```python
from build123d import *

# Parameters (mm, degrees)
SKETCH1_W           = 20.32
SKETCH1_H           = 26.081708108
SKETCH1_R           = 3.175
BOSS_EXTRUDE1_DEPTH = 22.098
SKETCH2_R           = 3.175
BOSS_EXTRUDE2_DEPTH = 5.08


with BuildPart() as part:
    # Sketch1 → Boss-Extrude1 (new body)
    with BuildSketch(Plane.XY):
        with Locations((-101.659894533, 115.530854428)):
            Rectangle(SKETCH1_W, SKETCH1_H)
        with Locations(Location((-104.04520642, 114, 0), (0, 0, 180))):
            Circle(SKETCH1_R, mode=Mode.SUBTRACT)
        with Locations(Location((-104.05047074, 124, 0), (0, 0, 180))):
            Circle(SKETCH1_R, mode=Mode.SUBTRACT)
    extrude(amount=BOSS_EXTRUDE1_DEPTH)

    # Sketch2 → Boss-Extrude2 (add)
    with BuildSketch(Plane(origin=(0, 102.490000374, 0), x_dir=(1, 0, 0), z_dir=(0, 1, 0))):
        Polygon((-96.663626928, 22.420429911), (-114.413437041, -43.822763256), (-93.559098452, -49.410666439), (-75.809288339, 16.832526727), align=None)
        with Locations(Location((-101.685366436, -38.029634252, 0), (0, 0, 270))):
            Circle(SKETCH2_R, mode=Mode.SUBTRACT)
        with Locations(Location((-88.537358944, 11.039397724, 0), (0, 0, 270))):
            Circle(SKETCH2_R, mode=Mode.SUBTRACT)
    extrude(amount=-BOSS_EXTRUDE2_DEPTH)


solid = part.part
```
The model under review builds one solid part; all positions refer to its coordinate system, in mm. A direction names the side the tool comes from. Coordinates: 2 decimals unless noted, no trailing zeros. Write each loop counter-clockwise with the first axis right and the second up, starting at its lowest first coordinate (ties: lowest second). Pieces come first, ordered by that corner, then holes. Notation, with made-up numbers: (52, -36) -> (67, -36) arc R35 cw to (67, 2) -> close; hole circle Ø4 at (-10, 12.5). An arc over 180 degrees is marked (long way). One line per item, written item: value. Start each with the question number.
Q1. To check wall thickness, follow probe 1 along X at (y, z) = (114, 16.5); probe 2 along Y at (x, z) = (-90.5, 36); probe 3 along Z at (x, y) = (-96.5, 116). State the ranges of each line that lie inside material, in increasing order.
Q2. Add section B-B, the plane z = 37. Give the boundary of the cut face in (x, y), then the cut area to 3 significant figures.
Q3. Clearance check with flat-ended pins moving along their axes: P1, Ø5, axis at x = -104.05, y = 124, coming from the -Z side; P2, Ø6.5, axis at y = 115, z = 9, coming from the -X side; P3, Ø12, axis at x = -90.5, y = 123.5, coming from the +Z side; P4, Ø5, axis at x = -93.5, y = 115, coming from the -Z side. State where each tip first meets the part, or that it passes through.
Q4. Add section D-D, the plane y = 107. Give the boundary of the cut face in (x, z), then the cut area to 3 significant figures.
Q5. For faces 1 (the face through (-100, 116, 0)), 2 (the face through (-100.732, 99.986, 41.058)), 3 (the face through (-108, 102.49, 8)), 4 (the face through (-91.5, 115, 11)), list the 3-axis set-ups (+Z, -Z, +X, -X, +Y, -Y) from which the entire face can be reached by the end or side of a thin tool; tool diameter is ignored.
Q6. The part is to be moulded in two halves that separate along Y. For faces 5 (the face through (-103.64, 120.85, 10.89)), 6 (the face through (-105.75, 111.32, 10.89)), 7 (the face through (-91, 102.49, 13)), 8 (the face through (-100, 116, 22.098)), say which applies: +Y half, -Y half, draft (parallel to the pull), parting line (faces both ways), or undercut.
Q7. Add section A-A, the plane y = 114. Give the boundary of the cut face in (x, z), then the cut area to 3 significant figures.
Q8. Add section C-C, the plane z = 10. Give the boundary of the cut face in (x, y) (3 decimals).
Response:
1. probe 1: -111.82 to -107.22, -100.87 to -91.5
1. probe 2: 97.41 to 102.49
1. probe 3: 0 to 22.1
2. outline: (-112.59, 97.41) -> (-104.69, 97.41) -> (-104.69, 102.49) -> (-112.59, 102.49) -> close; (-98.68, 97.41) -> (-90.23, 97.41) -> (-90.23, 102.49) -> (-98.68, 102.49) -> close
2. area: 83.0 mm²
3. P1: through
3. P2: x = -111.82
3. P3: z = 22.1
3. P4: z = 0
4. outline: (-111.82, 0) -> (-91.5, 0) -> (-91.5, 22.1) -> (-111.82, 22.1) -> close
4. area: 449 mm²
5. face 1: -Z, +X, -X, +Y
5. face 2: +Y, -Y
5. face 3: -Z, -X, -Y
5. face 4: +Z, -Z, +X, +Y
6. face 5: undercut
6. face 6: undercut
6. face 7: +Y half
6. face 8: draft
7. outline: (-111.82, 0) -> (-107.22, 0) -> (-107.22, 22.1) -> (-111.82, 22.1) -> close; (-100.87, 0) -> (-91.5, 0) -> (-91.5, 22.1) -> (-100.87, 22.1) -> close
7. area: 309 mm²
8. outline: (-111.82, 102.49) -> (-105.351, 102.49) -> (-105.351, 97.41) -> (-82.999, 97.41) -> (-82.999, 102.49) -> (-91.5, 102.49) -> (-91.5, 128.572) -> (-111.82, 128.572) -> close; hole circle Ø6.35 at (-104.05, 124); hole circle Ø6.35 at (-104.045, 114)
